```python
from build123d import *

# Parameters (mm, degrees)
SKETCH1_W             = 50.8
SKETCH1_H             = 76.2
BOSS_EXTRUDE1_DEPTH   = 100
SKETCH2_W             = 46.8
SKETCH2_H             = 72.2
CUT_EXTRUDE1_DEPTH    = 110.985317202
FILLET2_R             = 2
CORTAR_EXTRUIR2_DEPTH = 10
CROQUIS4_R            = 2.5
CORTAR_EXTRUIR5_DEPTH = 10
CROQUIS6_R            = 2.5
CORTAR_EXTRUIR6_DEPTH = 10


with BuildPart() as part:
    # Sketch1 → Boss-Extrude1 (new body)
    with BuildSketch(Plane(origin=(0, 0, 0), x_dir=(0, 0, -1), z_dir=(1, 0, 0))):
        Rectangle(SKETCH1_W, SKETCH1_H)
    extrude(amount=-BOSS_EXTRUDE1_DEPTH)

    # Sketch2 → Cut-Extrude1 (cut, through all)
    with BuildSketch(Plane(origin=(0, 0, 0), x_dir=(0, 0, -1), z_dir=(1, 0, 0))):
        Rectangle(SKETCH2_W, SKETCH2_H)
    extrude(amount=-CUT_EXTRUDE1_DEPTH, mode=Mode.SUBTRACT)

    # Fillet2
    fillet2_edges = [part.edges().sort_by_distance(p)[0] for p in [
        (-50, -36.1, 23.4),
        (-50, 36.1, 23.4),
        (-50, 36.1, -23.4),
        (-50, -36.1, -23.4),
        (-50, 38.1, 25.4),
        (-50, 38.1, -25.4),
        (-50, -38.1, -25.4),
        (-50, -38.1, 25.4),
    ]]
    fillet(fillet2_edges, radius=FILLET2_R)

    # Croquis2 → Cortar-Extruir2 (cut)
    with BuildSketch(Plane.XY.offset(25.4)):
        with BuildLine():
            ThreePointArc((-27, 26.5), (-30, 29.5), (-33, 26.5))
            Line((-33, 26.5), (-30, 26.5))
            Line((-30, 26.5), (-30, 23.5))
            ThreePointArc((-30, 23.5), (-27.878679656, 24.378679656), (-27, 26.5))
        make_face()
        with BuildLine():
            Line((-30, 26.5), (-33, 26.5))
            ThreePointArc((-33, 26.5), (-32.121320344, 24.378679656), (-30, 23.5))
            Line((-30, 23.5), (-30, 26.5))
        make_face()
        with BuildLine():
            ThreePointArc((-70, 23.5), (-67.878679656, 24.378679656), (-67, 26.5))
            Line((-67, 26.5), (-70, 26.5))
            Line((-70, 26.5), (-70, 23.5))
        make_face()
        with BuildLine():
            Line((-70, 26.5), (-67, 26.5))
            ThreePointArc((-67, 26.5), (-72.121320344, 28.621320344), (-70, 23.5))
            Line((-70, 23.5), (-70, 26.5))
        make_face()
        with BuildLine():
            ThreePointArc((-67, -26.5), (-67.878679656, -24.378679656), (-70, -23.5))
            Line((-70, -23.5), (-70, -26.5))
            Line((-70, -26.5), (-67, -26.5))
        make_face()
        with BuildLine():
            Line((-70, -26.5), (-70, -23.5))
            ThreePointArc((-70, -23.5), (-72.121320344, -28.621320344), (-67, -26.5))
            Line((-67, -26.5), (-70, -26.5))
        make_face()
        with BuildLine():
            ThreePointArc((-27, -26.5), (-27.878679656, -24.378679656), (-30, -23.5))
            Line((-30, -23.5), (-30, -26.5))
            Line((-30, -26.5), (-33, -26.5))
            ThreePointArc((-33, -26.5), (-30, -29.5), (-27, -26.5))
        make_face()
        with BuildLine():
            Line((-30, -26.5), (-30, -23.5))
            ThreePointArc((-30, -23.5), (-32.121320344, -24.378679656), (-33, -26.5))
            Line((-33, -26.5), (-30, -26.5))
        make_face()
    extrude(amount=-CORTAR_EXTRUIR2_DEPTH, mode=Mode.SUBTRACT)

    # Croquis4 → Cortar-Extruir5 (cut)
    with BuildSketch(Plane(origin=(0, 0, -25.4), x_dir=(-1, 0, 0), z_dir=(0, 0, -1))):
        with Locations(Location((90, 20, 0), (0, 0, 90))):
            Circle(CROQUIS4_R)
        with Locations(Location((59.2, 20, 0), (0, 0, 90))):
            Circle(CROQUIS4_R)
        with Locations(Location((59.2, -20, 0), (0, 0, 90))):
            Circle(CROQUIS4_R)
        with Locations(Location((90, -20, 0), (0, 0, 90))):
            Circle(CROQUIS4_R)
        with Locations(Location((74.6, 0, 0), (0, 0, 90))):
            Circle(CROQUIS4_R)
    extrude(amount=-CORTAR_EXTRUIR5_DEPTH, mode=Mode.SUBTRACT)

    # Croquis6 → Cortar-Extruir6 (cut)
    with BuildSketch(Plane(origin=(0, 0, -25.4), x_dir=(-1, 0, 0), z_dir=(0, 0, -1))):
        with Locations(Location((17.2, 20, 0), (0, 0, 90))):
            Circle(CROQUIS6_R)
        with Locations(Location((17.2, -20, 0), (0, 0, 90))):
            Circle(CROQUIS6_R)
        with Locations(Location((41.2, -20, 0), (0, 0, 90))):
            Circle(CROQUIS6_R)
        with Locations(Location((41.2, 20, 0), (0, 0, 90))):
            Circle(CROQUIS6_R)
    extrude(amount=-CORTAR_EXTRUIR6_DEPTH, mode=Mode.SUBTRACT)


solid = part.part
```
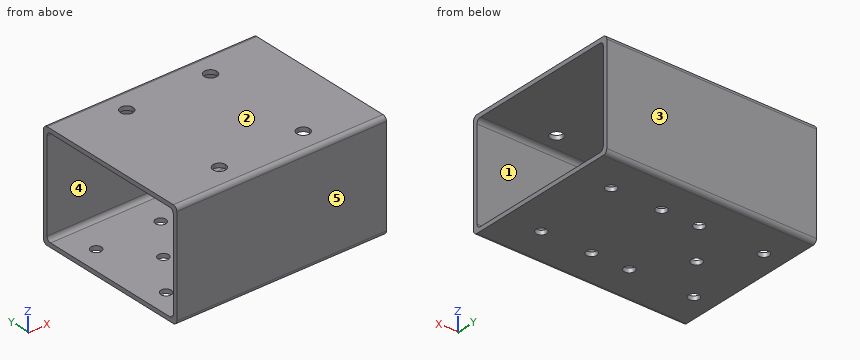
Geometry: final body of the model. Coordinates: model frame, mm. Face numbers are marked on the shaded views. A direction names the side the tool comes from. Round coordinates to 2 decimals unless told otherwise and drop trailing zeros. Write each loop counter-clockwise with the first axis right and the second up, starting at its lowest first coordinate (ties: lowest second). Pieces come first, ordered by that corner, then holes. Notation, with made-up numbers: M 83.25,81 L 140.25,81 A24 ccw 140.25,102 Z; hole C -6,-7 d7. An arc over 180 degrees is marked long. Answer in a Markdown table with one row per item. Add a question column.
(1) Cut plane D-D, the plane x = -59.2. Return the cut outline in (y, z), then the cut area to 3 significant figures.
(2) Ray query, L1, parallel to Y at x = -15, z = 21; L2, parallel to Z at x = -38.5, y = -29; L3, parallel to X at y = -20, z = -24.1. Return the intervals inside material, ascending.
(3) Reachability of the marked faces 1 and 2 from +Z, -Z, +X, -X, +Y, -Y: full face, straight path, thin tool, end or side. Return the list, or none.
(4) Cut plane A-A, the plane y = -15. Return the cut outline in (x, z), then the cut area to 3 significant figures.
(5) Cut plane B-B, the plane z = -5.5. Return the cut outline in (x, y), then the cut area to 3 significant figures.
(6) Contact query for flat-ended pins moving along their axis: pin 1 (3 mm diameter, centred on x = -41.2, y = -20, fed in from -Z); pin 2 (10 mm diameter, centred on y = 21.5, z = 17, fed in from -X). Output: stop coordinate, or through.
(7) Draft query along Y for the marked faces 3, 4 and 5. Return one class per face: pulls with the +Y half, pulls with the -Y half, needs draft (parallel to the pull), parting line crosses it, or undercut.
(8) Cut plane C-C, the plane x = -13. Return the cut outline in (y, z).
Established:
| question | item | result |
|---|---|---|
| 1 | outline | M -38.1,-23.4 A2 ccw -36.1,-25.4 L -22.5,-25.4 L -22.5,-23.4 L -34.1,-23.4 A2 cw -36.1,-21.4 L -36.1,21.4 A2 cw -34.1,23.4 L 34.1,23.4 A2 cw 36.1,21.4 L 36.1,-21.4 A2 cw 34.1,-23.4 L 22.5,-23.4 L 22.5,-25.4 L 36.1,-25.4 A2 ccw 38.1,-23.4 L 38.1,23.4 A2 ccw 36.1,25.4 L -36.1,25.4 A2 ccw -38.1,23.4 Z; M -17.5,-25.4 L 17.5,-25.4 L 17.5,-23.4 L -17.5,-23.4 Z |
| 1 | area | 472 mm² |
| 2 | L1 | -38.1 to -36.1, 36.1 to 38.1 |
| 2 | L2 | -25.4 to -23.4, 23.4 to 25.4 |
| 2 | L3 | -100 to -92.5, -87.5 to -61.7, -56.7 to -43.7, -38.7 to -19.7, -14.7 to 0 |
| 3 | face 1 | +X, -X |
| 3 | face 2 | +Z, +X, -X, +Y, -Y |
| 4 | outline | M -100,-25.4 L 0,-25.4 L 0,-23.4 L -100,-23.4 Z; M -100,23.4 L 0,23.4 L 0,25.4 L -100,25.4 Z |
| 4 | area | 400 mm² |
| 5 | outline | M -100,-38.1 L 0,-38.1 L 0,-36.1 L -100,-36.1 Z; M -100,36.1 L 0,36.1 L 0,38.1 L -100,38.1 Z |
| 5 | area | 400 mm² |
| 6 | pin 1 | z = 23.4 |
| 6 | pin 2 | through |
| 7 | face 3 | pulls with the +Y half |
| 7 | face 4 | undercut |
| 7 | face 5 | pulls with the -Y half |
| 8 | outline | M -38.1,-23.4 A2 ccw -36.1,-25.4 L 36.1,-25.4 A2 ccw 38.1,-23.4 L 38.1,23.4 A2 ccw 36.1,25.4 L -36.1,25.4 A2 ccw -38.1,23.4 Z; hole M -36.1,-21.4 A2 ccw -34.1,-23.4 L 34.1,-23.4 A2 ccw 36.1,-21.4 L 36.1,21.4 A2 ccw 34.1,23.4 L -34.1,23.4 A2 ccw -36.1,21.4 Z |
